from build123d import *
from OCP.BRepFilletAPI import BRepFilletAPI_MakeChamfer

# Parameters (mm, degrees)
SKETCH_1_W          = 12
SKETCH_1_H          = 46
EXTRUDE_1_DEPTH     = 59
SKETCH_2_W          = 20
SKETCH_2_H          = 46.080872769
CUT_EXTRUDE_1_DEPTH = 60
SKETCH_3_W          = 12
SKETCH_3_H          = 59
EXTRUDE_2_DEPTH     = 5
SKETCH_4_W          = 12
SKETCH_4_H          = 56
EXTRUDE_3_DEPTH     = 40
SKETCH_5_W          = 12
SKETCH_5_H          = 7
EXTRUDE_4_DEPTH     = 12
M4_A_1_D            = 4.5
M4_A_1_CBORE_D      = 10.705
M4_A_1_CBORE_DEPTH  = 2.8
SKETCH_8_W          = 15
SKETCH_8_H          = 56
EXTRUDE_5_DEPTH     = 3
SKETCH_9_W          = 6
SKETCH_9_H          = 40
CUT_EXTRUDE_2_DEPTH = 6
CHAMFER_1_SIZE      = 8
CHAMFER_1_SIZE_2    = 5.601660306
SKETCH_10_W         = 6
SKETCH_10_H         = 39.2
EXTRUDE_6_DEPTH     = 9
SKETCH_11_W         = 3
SKETCH_11_H         = 0.4
CUT_EXTRUDE_3_DEPTH = 119.330046903
CHAMFER_2_SIZE      = 1
CHAMFER_3_SIZE      = 2
CHAMFER_3_SIZE2     = 1.400415076
SKETCH_12_W         = 45
SKETCH_12_H         = 20.5
CUT_EXTRUDE_4_DEPTH = 4
SKETCH_14_W         = 7
SKETCH_14_H         = 80
EXTRUDE_7_DEPTH     = 10
CUT_EXTRUDE_5_DEPTH = 103.46950766
SKETCH_16_W         = 3
SKETCH_16_H         = 56
EXTRUDE_8_DEPTH     = 12
CHAMFER_5_SIZE      = 5
CUT_EXTRUDE_START   = -43.060641
SKETCH_17_W         = 3
SKETCH_17_H         = 56
CUT_EXTRUDE_6_DEPTH = 43.060641
CHAMFER_4_SIZE      = 1
FILLET_1_R          = 12
SKETCH_22_W         = 3
SKETCH_22_H         = 80
EXTRUDE_11_DEPTH    = 0.8
SKETCH_24_W         = 9
SKETCH_24_H         = 2
EXTRUDE_13_DEPTH    = 1
SKETCH_26_W         = 99
SKETCH_26_H         = 80
CUT_EXTRUDE_8_DEPTH = 0.4


with BuildPart() as part:
    # Sketch 1 → Extrude 1 (new body)
    with BuildSketch(Plane.XY):
        Rectangle(SKETCH_1_W, SKETCH_1_H)
    extrude(amount=EXTRUDE_1_DEPTH)

    # Sketch 2 → Cut-Extrude 1 (cut)
    with BuildSketch(Plane(origin=(6, 0, 0), x_dir=(0, 0, -1), z_dir=(1, 0, 0))):
        with Locations((-32, 0.040436385)):
            Rectangle(SKETCH_2_W, SKETCH_2_H)
    extrude(amount=-CUT_EXTRUDE_1_DEPTH, mode=Mode.SUBTRACT)


with BuildPart() as cut_extrude_1_piece_1:
    # of the separate pieces the step leaves, piece 1, a body of its own (cut_extrude_1_pieces)
    add(part.part.solids().sort_by_distance((-6, 23, 0))[0])



with BuildPart() as cut_extrude_1_piece_2:
    # of the separate pieces the step leaves, piece 2, a body of its own (cut_extrude_1_pieces)
    add(part.part.solids().sort_by_distance((6, 23, 42))[0])


with BuildPart() as cut_extrude_1_piece_1_1:
    add(cut_extrude_1_piece_1.part)

    add(cut_extrude_1_piece_2.part)  # Extrude 2 merges Cut-Extrude 1 piece 2
    # Sketch 3 → Extrude 2 (add)
    with BuildSketch(Plane.XZ.offset(23)):
        with Locations((0, 29.5)):
            Rectangle(SKETCH_3_W, SKETCH_3_H)
    extrude_2 = extrude(amount=EXTRUDE_2_DEPTH)

    # Mirror 1: Extrude 2 across plane
    add(extrude_2.mirror(Plane.ZX))

    # Sketch 4 → Extrude 3 (add)
    with BuildSketch(Plane(origin=(0, 0, 0), x_dir=(-1, 0, 0), z_dir=(0, 0, -1))):
        Rectangle(SKETCH_4_W, SKETCH_4_H)
    extrude(amount=EXTRUDE_3_DEPTH)

    # Sketch 5 → Extrude 4 (add)
    with BuildSketch(Plane.XZ.offset(28)):
        with Locations((0, -36.5)):
            Rectangle(SKETCH_5_W, SKETCH_5_H)
    extrude_4 = extrude(amount=EXTRUDE_4_DEPTH)

    # Mirror 2: Extrude 4 across plane
    add(extrude_4.mirror(Plane.ZX))

    # M4 _ _ _ _ _A _1 (through all)
    with Locations(Plane.XY.offset(-33)):
        with Locations((0, -34), (0, 34)):
            CounterBoreHole(M4_A_1_D / 2, M4_A_1_CBORE_D / 2, M4_A_1_CBORE_DEPTH)

    # Sketch 8 → Extrude 5 (add)
    with BuildSketch(Plane.XY.offset(59)):
        with Locations((-1.5, 0)):
            Rectangle(SKETCH_8_W, SKETCH_8_H)
    extrude(amount=EXTRUDE_5_DEPTH)

    # Sketch 9 → Cut-Extrude 2 (cut)
    with BuildSketch(Plane.XY.offset(62)):
        with Locations((3, 0)):
            Rectangle(SKETCH_9_W, SKETCH_9_H)
    extrude(amount=-CUT_EXTRUDE_2_DEPTH, mode=Mode.SUBTRACT)

    # Chamfer 1
    chamfer_1_edges_1 = [cut_extrude_1_piece_1_1.edges().sort_by_distance(p)[0] for p in [
        (0, 0, 62),
    ]]
    chamfer_1_side_1 = [cut_extrude_1_piece_1_1.faces().sort_by_distance(p)[0] for p in [
        (-0.112033206, 0, 62),
    ]]
    chamfer_1_edges_2 = [cut_extrude_1_piece_1_1.edges().sort_by_distance(p)[0] for p in [
        (3, 20, 62),
    ]]
    chamfer_1_side_2 = [cut_extrude_1_piece_1_1.faces().sort_by_distance(p)[0] for p in [
        (3, 20.112033206, 62),
    ]]
    chamfer_1_edges_3 = [cut_extrude_1_piece_1_1.edges().sort_by_distance(p)[0] for p in [
        (3, -20, 62),
    ]]
    chamfer_1_side_3 = [cut_extrude_1_piece_1_1.faces().sort_by_distance(p)[0] for p in [
        (3, -20.112033206, 62),
    ]]
    chamfer_1 = BRepFilletAPI_MakeChamfer(cut_extrude_1_piece_1_1.part.solid().wrapped)
    for e in chamfer_1_edges_1:
        chamfer_1.Add(CHAMFER_1_SIZE - 0.0001, CHAMFER_1_SIZE_2 - 0.0001, e.wrapped, chamfer_1_side_1[0].wrapped)
    for e in chamfer_1_edges_2:
        chamfer_1.Add(CHAMFER_1_SIZE - 0.0001, CHAMFER_1_SIZE_2 - 0.0001, e.wrapped, chamfer_1_side_2[0].wrapped)
    for e in chamfer_1_edges_3:
        chamfer_1.Add(CHAMFER_1_SIZE - 0.0001, CHAMFER_1_SIZE_2 - 0.0001, e.wrapped, chamfer_1_side_3[0].wrapped)
    add(Compound.cast(chamfer_1.Shape()), mode=Mode.REPLACE)  # a hair under: the kernel refuses the full size

    # Sketch 10 → Extrude 6 (add)
    with BuildSketch(Plane(origin=(0, 0, -40), x_dir=(-1, 0, 0), z_dir=(0, 0, -1))):
        with Locations((-3, 0)):
            Rectangle(SKETCH_10_W, SKETCH_10_H)
    extrude(amount=EXTRUDE_6_DEPTH)

    # Sketch 11 → Cut-Extrude 3 (cut, through all)
    with BuildSketch(Plane.XY.offset(62)):
        with Locations((-7.5, 27.8)):
            Rectangle(SKETCH_11_W, SKETCH_11_H)
        with Locations((-7.5, -27.8)):
            Rectangle(SKETCH_11_W, SKETCH_11_H)
    extrude(amount=-CUT_EXTRUDE_3_DEPTH, mode=Mode.SUBTRACT)


with BuildPart() as cut_extrude_3_kept_piece:
    # of the separate pieces the step leaves, the one the design keeps (cut_extrude_3_pieces_kept)
    add(cut_extrude_1_piece_1_1.part.solids().sort_by_distance((6, -27.9999, 62))[0])

    # Chamfer 2
    chamfer_2_edges = [cut_extrude_3_kept_piece.edges().sort_by_distance(p)[0] for p in [
        (-7.5, -27.6, 59),
        (-7.5, 27.6, 59),
    ]]
    chamfer(chamfer_2_edges, length=CHAMFER_2_SIZE)

    # Chamfer 3: one chamfer whose edges measure the first distance from different faces: ONE call of the kernel's chamfer builder (chamfer() names one face for all edges)
    chamfer_3_edges_1 = [cut_extrude_3_kept_piece.edges().sort_by_distance(p)[0] for p in [
        (6, 0, -49),
    ]]
    chamfer_3_side_1 = [cut_extrude_3_kept_piece.faces().sort_by_distance(p)[0] for p in [
        (6, 0, -1.052959329),
    ]]
    chamfer_3_edges_2 = [cut_extrude_3_kept_piece.edges().sort_by_distance(p)[0] for p in [
        (3, -19.6, -49),
    ]]
    chamfer_3_side_2 = [cut_extrude_3_kept_piece.faces().sort_by_distance(p)[0] for p in [
        (3, -19.6, -44.5),
    ]]
    chamfer_3_edges_3 = [cut_extrude_3_kept_piece.edges().sort_by_distance(p)[0] for p in [
        (0, 0, -49),
    ]]
    chamfer_3_side_3 = [cut_extrude_3_kept_piece.faces().sort_by_distance(p)[0] for p in [
        (0, 0, -44.5),
    ]]
    chamfer_3_edges_4 = [cut_extrude_3_kept_piece.edges().sort_by_distance(p)[0] for p in [
        (3, 19.6, -49),
    ]]
    chamfer_3_side_4 = [cut_extrude_3_kept_piece.faces().sort_by_distance(p)[0] for p in [
        (3, 19.6, -44.5),
    ]]
    chamfer_3 = BRepFilletAPI_MakeChamfer(cut_extrude_3_kept_piece.part.solid().wrapped)
    for e in chamfer_3_edges_1:
        chamfer_3.Add(CHAMFER_3_SIZE, CHAMFER_3_SIZE2, e.wrapped, chamfer_3_side_1[0].wrapped)  # the first distance lies on this face
    for e in chamfer_3_edges_2:
        chamfer_3.Add(CHAMFER_3_SIZE, CHAMFER_3_SIZE2, e.wrapped, chamfer_3_side_2[0].wrapped)  # the first distance lies on this face
    for e in chamfer_3_edges_3:
        chamfer_3.Add(CHAMFER_3_SIZE, CHAMFER_3_SIZE2, e.wrapped, chamfer_3_side_3[0].wrapped)  # the first distance lies on this face
    for e in chamfer_3_edges_4:
        chamfer_3.Add(CHAMFER_3_SIZE, CHAMFER_3_SIZE2, e.wrapped, chamfer_3_side_4[0].wrapped)  # the first distance lies on this face
    add(Compound.cast(chamfer_3.Shape()), mode=Mode.REPLACE)

    # Sketch 12 → Cut-Extrude 4 (cut)
    with BuildSketch(Plane.ZY.offset(6)):
        with Locations((-5.5, 12.75)):
            Rectangle(SKETCH_12_W, SKETCH_12_H)
        with Locations((-5.5, -12.75)):
            Rectangle(SKETCH_12_W, SKETCH_12_H)
    cut_extrude_4 = extrude(amount=-CUT_EXTRUDE_4_DEPTH, mode=Mode.SUBTRACT)

    # Mirror 3: Cut-Extrude 4 across plane
    add(cut_extrude_4.mirror(Plane.ZY), mode=Mode.SUBTRACT)

    # Sketch 14 → Extrude 7 (add)
    with BuildSketch(Plane(origin=(6, 0, 0), x_dir=(0, 0, -1), z_dir=(1, 0, 0))):
        with Locations((36.5, 0)):
            Rectangle(SKETCH_14_W, SKETCH_14_H)
    extrude(amount=EXTRUDE_7_DEPTH)

    # Sketch 15 → Cut-Extrude 5 (cut, through all)
    with BuildSketch(Plane.XZ.offset(40)):
        with BuildLine():
            Line((6, -33), (16, -33))
            Line((16, -33), (16, -28.353890031))
            add(Edge.make_bspline(
                [(6, -33), (5.579283, -24.005465365), (9.542787604, -28.181394392), (15.145388019, -28.353890031), (16, -28.353890031)],
                knots=[0, 0, 0, 0, 0.752787833, 1, 1, 1, 1], degree=3))
        make_face()
    extrude(amount=-CUT_EXTRUDE_5_DEPTH, mode=Mode.SUBTRACT)

    # Sketch 16 → Extrude 8 (add)
    with BuildSketch(Plane(origin=(6, 0, 0), x_dir=(0, 0, -1), z_dir=(1, 0, 0))):
        with Locations((-17.43935887, 0)):
            Rectangle(SKETCH_16_W, SKETCH_16_H)
    extrude(amount=EXTRUDE_8_DEPTH)

    # Chamfer 5
    chamfer_5_edges = [cut_extrude_3_kept_piece.edges().sort_by_distance(p)[0] for p in [
        (16, 0, -33),
    ]]
    chamfer(chamfer_5_edges, length=CHAMFER_5_SIZE)

    # Sketch 17 → Cut-Extrude 6 (cut)
    with BuildSketch(Plane.XY.offset(62).offset(CUT_EXTRUDE_START)):
        with Locations((4.5, 0)):
            Rectangle(SKETCH_17_W, SKETCH_17_H)
    extrude(amount=CUT_EXTRUDE_6_DEPTH, mode=Mode.SUBTRACT)

    # Chamfer 4
    chamfer_4_edges = [cut_extrude_3_kept_piece.edges().sort_by_distance(p)[0] for p in [
        (3, -23, 32),
        (3, 23, 32),
        (3, 0, 22),
        (3, 0, 42),
    ]]
    chamfer(chamfer_4_edges, length=CHAMFER_4_SIZE)

    # Fillet 1
    fillet_1_edges = [cut_extrude_3_kept_piece.edges().sort_by_distance(p)[0] for p in [
        (6, -25.5, 15.93935887),
        (6, 0, 15.93935887),
        (6, 25.5, 15.93935887),
    ]]
    fillet(fillet_1_edges, radius=FILLET_1_R - 0.0001)  # a hair under: the kernel refuses the full size

    # Sketch 22 → Extrude 11 (add)
    with BuildSketch(Plane(origin=(0, 0, -40), x_dir=(-1, 0, 0), z_dir=(0, 0, -1))):
        with Locations((-14.5, 0)):
            Rectangle(SKETCH_22_W, SKETCH_22_H)
    extrude(amount=EXTRUDE_11_DEPTH)

    # Sketch 24 → Extrude 13 (add)
    with BuildSketch(Plane(origin=(0, 28, 0), x_dir=(1, 0, 0), z_dir=(0, 1, 0))):
        with Locations((-1.5, -61)):
            Rectangle(SKETCH_24_W, SKETCH_24_H)
    extrude_13 = extrude(amount=EXTRUDE_13_DEPTH)

    # Mirror 4: Extrude 13 across plane
    add(extrude_13.mirror(Plane.ZX))

    # Sketch 26 → Cut-Extrude 8 (cut)
    with BuildSketch(Plane.ZY.offset(6)):
        with Locations((9.5, 0)):
            Rectangle(SKETCH_26_W, SKETCH_26_H)
    extrude(amount=-CUT_EXTRUDE_8_DEPTH, mode=Mode.SUBTRACT)


solid = cut_extrude_3_kept_piece.part
The model under review builds one solid part; all positions refer to its coordinate system, in mm. A direction names the side the tool comes from. Round coordinates to 2 decimals unless told otherwise and drop trailing zeros. Loops run counter-clockwise (first coordinate to the right, second up) from the corner with the lowest first, then second, coordinate; pieces in that order, holes last. Notation, with made-up numbers: (41, -11) -> (80, -11) arc R9 ccw to (80, 6) -> close; hole circle Ø4 at (-9.75, 67.5). An arc over 180 degrees is marked (long way). Return JSON: item names as keys, results as strings.
(1) For pin 1 (1 mm diameter, centred on x = 15, y = 13.5, fed in from +Z); pin 2 (12 mm diameter, centred on x = 6.5, z = -24.5, fed in from -Y); pin 3 (0.8 mm diameter, centred on x = -3.5, y = 28.5, fed in from -Z); pin 4 (12 mm diameter, centred on x = -1, y = -34.5, fed in from +Z), all flat-tipped, find the tip position at first contact; note any pin that passes through.
Solved:
{"pin 1": "z = 18.94", "pin 2": "y = -28", "pin 3": "z = -40", "pin 4": "z = 62"}
(2) Add section A-A on y = -34. Write out the cut boundary in (x, z).
Solved:
{"outline": "(-5.6, -40) -> (-2.25, -40) -> (-2.25, -35.8) -> (-5.35, -35.8) -> (-5.35, -33) -> (-5.6, -33) -> close; (2.25, -40) -> (13, -40) -> (13, -40.8) -> (16, -40.8) -> (16, -38) -> (11, -33) -> (5.35, -33) -> (5.35, -35.8) -> (2.25, -35.8) -> close"}
(3) For line 1 (Y direction, x = 0, z = -37.55); line 2 (Y direction, x = 0, z = -34.15); line 3 (Z direction, x = -2.25, y = 13), list the stretches that pass through material, from the lowest coordinate up.
Solved:
{"line 1": "-40 to -36.25, -31.75 to 31.75, 36.25 to 40", "line 2": "-40 to -39.35, -28.65 to 28.65, 39.35 to 40", "line 3": "-40 to -28, 17 to 22, 42 to 57.97"}
(4) The part is to be moulded in two halves that separate along Z. For faces 1 (the flat face through (-7, 0, 59)), 2 (the flat face through (-4, 23, -6)), 3 (the flat face through (-6, 28, 61)), say which applies: released by +Z, released by -Z, zero draft, split by the parting line, or undercut.
Solved:
{"face 1": "released by -Z", "face 2": "undercut", "face 3": "zero draft"}
(5) For faces 4 (the cylindrical face through (9.42, 25.54, 12.33)), 5 (the flat face through (4, 13, 17)), 6 (the flat face through (-4, -13, 17)), 7 (the flat face through (-1.2, 24.83, 59.78)), list the 3-axis set-ups (+Z, -Z, +X, -X, +Y, -Y) from which the entire face can be reached by the end or side of a thin tool; tool diameter is ignored.
Solved:
{"face 4": "+X, +Y, -Y", "face 5": "none", "face 6": "-X", "face 7": "+Z, +X"}
(6) Add section B-B on x = 8.25. Write out the cut boundary in (y, z).
Solved:
{"outline": "(-40, -40) -> (40, -40) -> (40, -33) -> (-40, -33) -> close; (-28, 10.93) -> (-23, 10.93) -> (-23, 15.94) -> (-2.5, 15.94) -> (-2.5, 10.93) -> (2.5, 10.93) -> (2.5, 15.94) -> (23, 15.94) -> (23, 10.93) -> (28, 10.93) -> (28, 18.94) -> (-28, 18.94) -> close"}
(7) Add section D-D on z = 14. Write out the cut boundary in (x, y), plus the area to 3 significant figures.
Solved:
{"outline": "(-5.6, -28) -> (11.46, -28) -> (11.46, -23) -> (2, -23) -> (2, -2.5) -> (11.46, -2.5) -> (11.46, 2.5) -> (2, 2.5) -> (2, 23) -> (11.46, 23) -> (11.46, 28) -> (-5.6, 28) -> (-5.6, 23) -> (-2, 23) -> (-2, 2.5) -> (-5.6, 2.5) -> (-5.6, -2.5) -> (-2, -2.5) -> (-2, -23) -> (-5.6, -23) -> close", "area": "420 mm2"}
(8) Add section C-C on z = -3. Write out the cut boundary in (x, y).
Solved:
{"outline": "(-5.6, -28) -> (6, -28) -> (6, -23) -> (2, -23) -> (2, -2.5) -> (6, -2.5) -> (6, 2.5) -> (2, 2.5) -> (2, 23) -> (6, 23) -> (6, 28) -> (-5.6, 28) -> (-5.6, 23) -> (-2, 23) -> (-2, 2.5) -> (-5.6, 2.5) -> (-5.6, -2.5) -> (-2, -2.5) -> (-2, -23) -> (-5.6, -23) -> close"}
